Could you check a few things on this model? Use its own coordinates, in mm. Give positions to 0.01 mm unless a question says otherwise; leave off trailing zeros. Loops run counter-clockwise (first coordinate to the right, second up) from the corner with the lowest first, then second, coordinate; pieces in that order, holes last. Notation, with made-up numbers: (45.5, 24.25) -> (67.5, 24.25) arc R11 ccw to (67.5, 42.25) -> close; hole circle Ø10 at (-15, 12). An arc over 180 degrees is marked (long way). Write item = value, one per line. Start each with the question number.
1) I want a section at A-A (y = 10.61). List the corners of the cut face in (x, z) for me (3 decimals).
2) I'm going to push flat-ended pins straight in: pin 1 Ø1 at (x, y) = (8.45, 20.925) entering from +Z; pin 2 Ø0.7 at (y, z) = (1.5, 1) entering from -X. Where does each tip first touch, or does it pass through?
3) I want a section at B-B (z = 0.5). Count the separate pieces of the cut face and the enclosed holes in it, and give its area (3 significant figures).
4) I need wall thicknesses on probe 1 along Y at (x, z) = (29, 0.3); probe 2 along X at (y, z) = (39, 0.95); probe 3 along Y at (x, z) = (8.45, 1.3) (3 decimals). Which ranges of each line are inside material? Lowest first, please. Write a range as from..to.
from build123d import *

# Parameters (mm, degrees)
SKETCH_1_R      = 1.1
SKETCH_1_R_2    = 0.45
SKETCH_1_R_3    = 0.325
SKETCH_1_R_4    = 0.8
SKETCH_1_R_5    = 0.4
SKETCH_1_R_6    = 1.099998
EXTRUDE_1_DEPTH = 1.6


with BuildPart() as part:
    # 草图1 → 凸台-拉伸1 (new body)
    with BuildSketch(Plane(origin=(0, 0, 0), x_dir=(-1, 0, 0), z_dir=(0, 0, -1))):
        with BuildLine():
            Line((-28.92416249, 0.002948493), (-3.030002484, 0.0047195))
            ThreePointArc((-3.030002484, 0.0047195), (-1.293435555, 0.73352407), (-0.582919351, 2.477653515))
            Line((-0.582919351, 2.477653515), (-0.581684294, 44.468735287))
            ThreePointArc((-0.581684294, 44.468735287), (-1.306942661, 46.21181505), (-3.054644493, 46.925863413))
            Line((-3.054644493, 46.925863413), (-28.9511375, 46.920055471))
            ThreePointArc((-28.9511375, 46.920055471), (-30.694165746, 46.194778446), (-31.408188877, 44.447109943))
            Line((-31.408188877, 44.447109943), (-31.397105, 2.460002))
            ThreePointArc((-31.397105, 2.460002), (-30.671824776, 0.716978502), (-28.92416249, 0.002948493))
        make_face()
        with Locations(Location((-28.94, 2.662946, 0), (0, 0, 180))):
            Circle(SKETCH_1_R, mode=Mode.SUBTRACT)
        with Locations(Location((-29.855, 7.61, 0), (0, 0, 180))):
            Circle(SKETCH_1_R_2, mode=Mode.SUBTRACT)
        with Locations(Location((-29.855, 10.61, 0), (0, 0, 180))):
            Circle(SKETCH_1_R_2, mode=Mode.SUBTRACT)
        with Locations(Location((-18.384, 5.145, 0), (0, 0, 180))):
            Circle(SKETCH_1_R_3, mode=Mode.SUBTRACT)
        with Locations(Location((-12.604, 5.145, 0), (0, 0, 180))):
            Circle(SKETCH_1_R_3, mode=Mode.SUBTRACT)
        with Locations(Location((-3.136974, 2.65, 0), (0, 0, 180))):
            Circle(SKETCH_1_R, mode=Mode.SUBTRACT)
        with Locations(Location((-8.45, 20.925, 0), (0, 0, 180))):
            Circle(SKETCH_1_R_4, mode=Mode.SUBTRACT)
        with Locations(Location((-30.15, 35.08, 0), (0, 0, 180))):
            Circle(SKETCH_1_R_5, mode=Mode.SUBTRACT)
        with Locations(Location((-30.15, 37.08, 0), (0, 0, 180))):
            Circle(SKETCH_1_R_5, mode=Mode.SUBTRACT)
        with Locations(Location((-28.15, 35.08, 0), (0, 0, 180))):
            Circle(SKETCH_1_R_5, mode=Mode.SUBTRACT)
        with Locations(Location((-28.15, 37.08, 0), (0, 0, 180))):
            Circle(SKETCH_1_R_5, mode=Mode.SUBTRACT)
        with Locations(Location((-30.15, 39.08, 0), (0, 0, 180))):
            Circle(SKETCH_1_R_5, mode=Mode.SUBTRACT)
        with Locations(Location((-28.15, 39.08, 0), (0, 0, 180))):
            Circle(SKETCH_1_R_5, mode=Mode.SUBTRACT)
        with Locations(Location((-30.15, 41.08, 0), (0, 0, 180))):
            Circle(SKETCH_1_R_5, mode=Mode.SUBTRACT)
        with Locations(Location((-28.15, 41.08, 0), (0, 0, 180))):
            Circle(SKETCH_1_R_5, mode=Mode.SUBTRACT)
        with Locations(Location((-28.951135, 44.462946, 0), (0, 0, 180))):
            Circle(SKETCH_1_R, mode=Mode.SUBTRACT)
        with Locations(Location((-8.45, 26.925, 0), (0, 0, 180))):
            Circle(SKETCH_1_R_4, mode=Mode.SUBTRACT)
        with Locations(Location((-3.038791293, 44.468807556, 0), (0, 0, 180))):
            Circle(SKETCH_1_R_6, mode=Mode.SUBTRACT)
        with BuildLine():
            Line((-19.514, 1.765), (-19.514, 1.165))
            ThreePointArc((-19.514, 1.165), (-19.814, 0.865), (-20.114, 1.165))
            Line((-20.114, 1.165), (-20.114, 1.765))
            ThreePointArc((-20.114, 1.765), (-19.814, 2.065), (-19.514, 1.765))
        make_face(mode=Mode.SUBTRACT)
        with BuildLine():
            Line((-19.514, 6.195), (-19.514, 5.095))
            ThreePointArc((-19.514, 5.095), (-19.814, 4.795), (-20.114, 5.095))
            Line((-20.114, 5.095), (-20.114, 6.195))
            ThreePointArc((-20.114, 6.195), (-19.814, 6.495), (-19.514, 6.195))
        make_face(mode=Mode.SUBTRACT)
        with BuildLine():
            Line((-10.874, 1.765), (-10.874, 1.165))
            ThreePointArc((-10.874, 1.165), (-11.174, 0.865), (-11.474, 1.165))
            Line((-11.474, 1.165), (-11.474, 1.765))
            ThreePointArc((-11.474, 1.765), (-11.174, 2.065), (-10.874, 1.765))
        make_face(mode=Mode.SUBTRACT)
        with BuildLine():
            Line((-10.874, 6.195), (-10.874, 5.095))
            ThreePointArc((-10.874, 5.095), (-11.174, 4.795), (-11.474, 5.095))
            Line((-11.474, 5.095), (-11.474, 6.195))
            ThreePointArc((-11.474, 6.195), (-11.174, 6.495), (-10.874, 6.195))
        make_face(mode=Mode.SUBTRACT)
    extrude(amount=-EXTRUDE_1_DEPTH)


solid = part.part
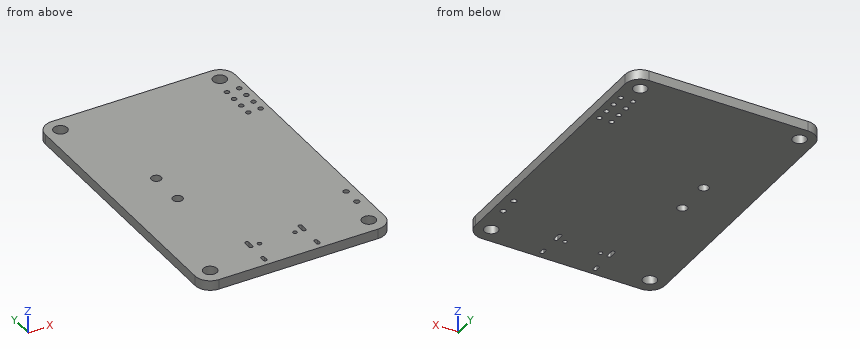
Answer list:
q1.outline = (0.583, 0) -> (29.405, 0) -> (29.405, 1.6) -> (0.583, 1.6) -> close; (30.305, 0) -> (31.399, 0) -> (31.399, 1.6) -> (30.305, 1.6) -> close
q2.pin_1 = through
q2.pin_2 = 0.66
q3.separate_pieces = 1
q3.enclosed_holes = 22
q3.area = 1,410 mm^2
q4.probe_1 = 0..1.56, 3.76..43.36, 45.56..46.92
q4.probe_2 = 0.58..27.76, 28.54..29.76, 30.54..31.41
q4.probe_3 = 0.004..20.125, 21.725..26.125, 27.725..46.925
